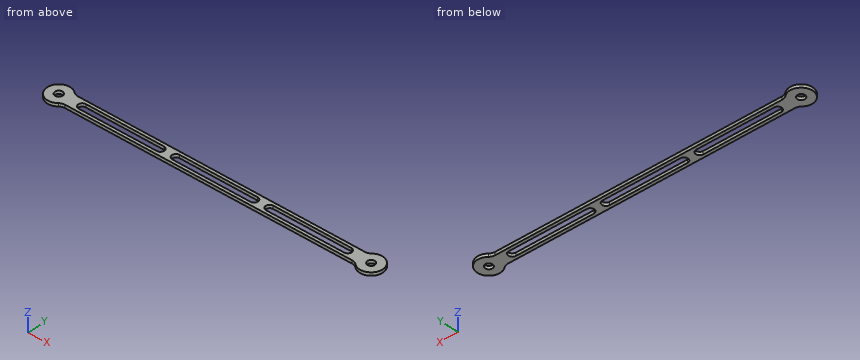
from build123d import *

# Parameters (mm, degrees)
SKETCH1_R           = 7.5
SKETCH1_R_2         = 2.45
SKETCH1_R_3         = 2.4
SKETCH1_W           = 188.02
SKETCH1_H           = 9
BOSS_EXTRUDE1_DEPTH = 2
CUT_EXTRUDE1_DEPTH  = 208.665115992
FILLET1_R           = 5


with BuildPart() as part:
    # Sketch1 → Boss-Extrude1 (new body)
    # profile 1 of 3: a face of its own
    with BuildSketch(Plane.XY):
        Circle(SKETCH1_R)
        Circle(SKETCH1_R_2, mode=Mode.SUBTRACT)
    # profile 2 of 3: a face of its own
    with BuildSketch(Plane.XY):
        with Locations((200.02, 0)):
            Circle(SKETCH1_R)
        with Locations((200.02, 0)):
            Circle(SKETCH1_R_3, mode=Mode.SUBTRACT)
    # profile 3 of 3: a face of its own
    with BuildSketch(Plane.XY):
        with Locations((100.01, 0)):
            Rectangle(SKETCH1_W, SKETCH1_H)
    extrude(amount=BOSS_EXTRUDE1_DEPTH)

    # Sketch2 → Cut-Extrude1 (cut, through all)
    with BuildSketch(Plane.XY.offset(2)):
        with BuildLine():
            Line((75, 2.5), (125, 2.5))
            ThreePointArc((125, 2.5), (127.5, 0), (125, -2.5))
            Line((125, -2.5), (75, -2.5))
            ThreePointArc((75, -2.5), (72.5, 0), (75, 2.5))
        make_face()
        with BuildLine():
            Line((135, 2.5), (185, 2.5))
            ThreePointArc((185, 2.5), (187.5, 0), (185, -2.5))
            Line((185, -2.5), (135, -2.5))
            ThreePointArc((135, -2.5), (132.5, 0), (135, 2.5))
        make_face()
        with BuildLine():
            Line((15, 2.5), (65, 2.5))
            ThreePointArc((65, 2.5), (67.5, 0), (65, -2.5))
            Line((65, -2.5), (15, -2.5))
            ThreePointArc((15, -2.5), (12.5, 0), (15, 2.5))
        make_face()
    extrude(amount=-CUT_EXTRUDE1_DEPTH, mode=Mode.SUBTRACT)

    # Fillet1
    fillet1_edges = [part.edges().sort_by_distance(p)[0] for p in [
        (6, -4.5, 1),
        (6, 4.5, 1),
        (194.02, 4.5, 1),
        (194.02, -4.5, 1),
    ]]
    fillet(fillet1_edges, radius=FILLET1_R)


solid = part.part
Here's how the part is built. I have some questions about the finished solid (model axes, mm). Give positions to 0.01 mm unless a question says otherwise; leave off trailing zeros. Order: outer loops, then holes, each group sorted by start corner. A loop starts at its lowest first (then second) coordinate and runs counter-clockwise, first axis right, second up. Notation, with made-up numbers: (-35.5, 18) -> (-4.5, 18) arc R32 cw to (-4.5, 53) -> close; hole circle Ø9 at (-15.5, -17.5). An arc over 180 degrees is marked (long way). One line per item, written item: value. Start each with the question number.
1. Imagine slicing it at A-A, the plane x = 0. List the corners of the cut face in (y, z) for me, plus the area to 3 significant figures.
2. I need wall thicknesses on probe 1 along Y at (x, z) = (161.5, 0.1); probe 2 along Y at (x, z) = (0, 1); probe 3 along X at (y, z) = (1, 1.25). Which ranges of each line are inside material? Lowest first, please. Write a range as from..to.
3. Imagine slicing it at B-B, the plane z = 0.5. List the corners of the cut face in (x, y) for me.
4. Imagine slicing it at C-C, the plane x = 200.02. List the corners of the cut face in (y, z) for me.
5. Will these pins go through, and if not, where does the flat tip stop? pin 1 Ø0.6 at (x, z) = (157.5, 0.5) entering from -Y; pin 2 Ø0.6 at (x, z) = (101.5, 1.5) entering from +Y; pin 3 Ø1 at (y, z) = (2, 1.5) entering from +X.
Values follow:
1. outline: (-7.5, 0) -> (-2.45, 0) -> (-2.45, 2) -> (-7.5, 2) -> close; (2.45, 0) -> (7.5, 0) -> (7.5, 2) -> (2.45, 2) -> close
1. area: 20.2 mm2
2. probe 1: y = -4.5..-2.5, 2.5..4.5
2. probe 2: y = -7.5..-2.45, 2.45..7.5
2. probe 3: x = -7.43..-2.24, 2.24..12.71, 67.29..72.71, 127.29..132.71, 187.29..197.84, 202.2..207.45
3. outline: (4.87, -5.7) arc R5 cw to (8.12, -4.5) -> (191.9, -4.5) arc R5 cw to (195.15, -5.7) arc R7.5 ccw (long way) to (195.15, 5.7) arc R5 cw to (191.9, 4.5) -> (8.12, 4.5) arc R5 cw to (4.87, 5.7) arc R7.5 ccw (long way) to start; hole circle Ø4.9 at (0, 0); hole (15, -2.5) -> (65, -2.5) arc R2.5 ccw to (65, 2.5) -> (15, 2.5) arc R2.5 ccw to start; hole (75, -2.5) -> (125, -2.5) arc R2.5 ccw to (125, 2.5) -> (75, 2.5) arc R2.5 ccw to start; hole (135, -2.5) -> (185, -2.5) arc R2.5 ccw to (185, 2.5) -> (135, 2.5) arc R2.5 ccw to start; hole circle Ø4.8 at (200.02, 0)
4. outline: (-7.5, 0) -> (-2.4, 0) -> (-2.4, 2) -> (-7.5, 2) -> close; (2.4, 0) -> (7.5, 0) -> (7.5, 2) -> (2.4, 2) -> close
5. pin 1: stops at y = -4.5
5. pin 2: stops at y = 4.5
5. pin 3: stops at x = 207.37
